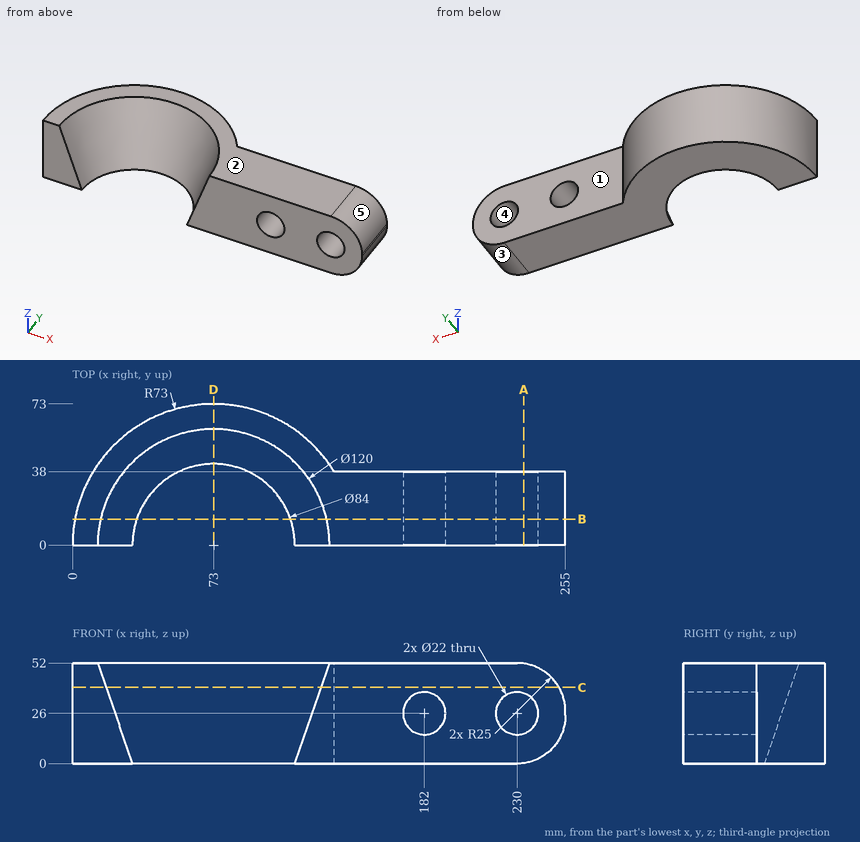
Geometry: see drawing. Coordinates: mm, zero at the bounding-box minimum. A direction names the side the tool comes from. Give positions to 0.01 mm unless a question says otherwise; leave off trailing zeros. Loops run counter-clockwise (first coordinate to the right, second up) from the corner with the lowest first, then second, coordinate; pieces in that order, holes last. Notation, with made-up numbers: (88.5, -15.5) -> (120.5, -15.5) arc R36 cw to (120.5, 19.5) -> close; hole circle Ø7 at (-24.75, 83.5). An arc over 180 degrees is marked (long way). Use one line per item in the form item = value.
Item 1: Section query C-C on z = 39.5. Output: boundary loops of the cut face in (x, y), and give its area (3 significant figures).
A:
outline = (0, 0) -> (17.33, 0) arc R55.67 cw to (128.67, 0) -> (251.65, 0) -> (251.65, 38) -> (135.33, 38) arc R73 ccw to start
area = 7,650 mm^2
Item 2: Section query B-B on y = 13.5. Give the number of separate pieces and of enclosed holes in the cut face, and give its area (3 significant figures).
A:
separate_pieces = 2
enclosed_holes = 2
area = 7,050 mm^2
Item 3: Access query for the marked faces 1 and 2. Directions: +Z, -Z, +X, -X, +Y, -Y. A direction counts if a zero-diameter tool reaches every point of the face in a straight line with its end or side. Return the directions, or none.
A:
face_1 = +Z, -Z, +X, +Y
face_2 = +Z, +X, -X, +Y, -Y
Item 4: Pin query (flat end, axial travel): P1, Ø10, axis at x = 39, z = 31, coming from the -Y side; P2, Ø12, axis at x = 140.5, z = 16, coming from the +Y side; P3, Ø10, axis at x = 74.5, z = 7.5, coming from the -Y side; P4, Ø5, axis at x = 188.5, z = 25, coming from the -Y side. Return the tip coordinate at first contact, or that it passes through.
A:
P1 = 34.92
P2 = 39.33
P3 = 42.83
P4 = through
Item 5: Line query: probe 1 along Z at (x, y) = (182, 30); probe 2 along X at (y, z) = (37.5, 20); probe 3 along X at (y, z) = (37, 19). Output: solid intervals per line, ascending.
A:
probe_1 = 0 to 15, 37 to 52
probe_2 = 10.37 to 41.58, 104.42 to 172.78, 191.22 to 220.78, 239.22 to 254.49
probe_3 = 10.07 to 41.52, 104.48 to 173.51, 190.49 to 221.51, 238.49 to 254.27
Item 6: Section query D-D on x = 73. Output: boundary loops of the cut face in (y, z).
A:
outline = (42, 0) -> (73, 0) -> (73, 52) -> (60, 52) -> close
Item 7: Draft query along Z for the marked faces 3, 4 and 5. Return one class per face: pulls with the +Z half, pulls with the -Z half, needs draft (parallel to the pull), parting line crosses it, or undercut.
A:
face_3 = pulls with the -Z half
face_4 = undercut
face_5 = pulls with the +Z half
Item 8: Section query A-A on x = 233.5. Output: boundary loops of the cut face in (y, z).
A:
outline = (0, 0.25) -> (38, 0.25) -> (38, 15.57) -> (0, 15.57) -> close; (0, 36.43) -> (38, 36.43) -> (38, 51.75) -> (0, 51.75) -> close
